Model file for the job. Use its own axes, mm. Round coordinates to 2 decimals unless told otherwise and drop trailing zeros. Write each loop counter-clockwise with the first axis right and the second up, starting at its lowest first coordinate (ties: lowest second). Pieces come first, ordered by that corner, then holes. Notation, with made-up numbers: (39.5, 30.25) - (67.5, 30.25) arc R5 cw to (67.5, 34.25) - close; hole circle Ø7 at (-19, 33). An arc over 180 degrees is marked (long way). One line per item, written item: value.
from build123d import *

# Parameters (mm, degrees)
SKETCH1_R           = 1.25
BOSS_EXTRUDE1_DEPTH = 3.9


with BuildPart() as part:
    # Sketch1 → Boss-Extrude1 (new body)
    with BuildSketch(Plane(origin=(0, 0, 0), x_dir=(1, 0, 0), z_dir=(0, 1, 0))):
        Polygon((-100, 14), (-125, 14), (-125, 5), (-121.1, 5), (-121.1, -5), (-125, -5), (-125, -14), (-60, -14), (-60, 3.5), (60, 3.5), (60, -14), (125, -14), (125, -5), (121.1, -5), (121.1, 5), (125, 5), (125, 14), (100, 14), (100, 17.9), (80, 17.9), (80, 14), (10, 14), (10, 17.9), (-10, 17.9), (-10, 14), (-80, 14), (-80, 17.9), (-100, 17.9), align=None)
        with Locations((-87.5, -9)):
            Circle(SKETCH1_R, mode=Mode.SUBTRACT)
        with Locations((87.5, -9)):
            Circle(SKETCH1_R, mode=Mode.SUBTRACT)
    extrude(amount=BOSS_EXTRUDE1_DEPTH)


solid = part.part
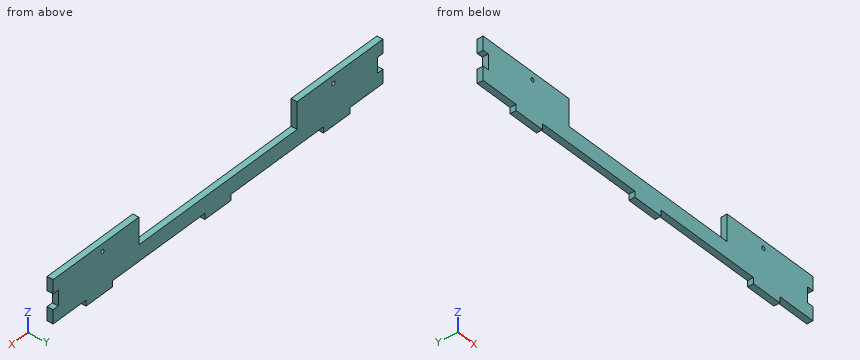
1. Band-saw the part on B-B on x = 43. Write the cut outline in (y, z), plus the area to 4 significant figures.
Report:
outline: (0, -14) - (3.9, -14) - (3.9, -3.5) - (0, -3.5) - close
area: 40.95 mm²
2. Drop flat-ended pins along their axis: pin 1 (1.2 mm diameter, centred on x = -116.5, y = 2.5, fed in from -Z); pin 2 (2 mm diameter, centred on x = -87.5, z = 9, fed in from -Y); pin 3 (5 mm diameter, centred on x = -63.5, z = -5.5, fed in from -Y); pin 4 (2 mm diameter, centred on y = 2.5, z = 0.5, fed in from +X). Give the stop position or say it passes through.
Report:
pin 1: z = -14
pin 2: through
pin 3: y = 0
pin 4: x = 121.1
3. Band-saw the part on A-A on y = 3.3. State how many separate pieces and enclosed holes the cut face has, plus the area to 3 significant figures.
Report:
separate pieces: 1
enclosed holes: 2
area: 5,050 mm²
4. Wall check: probe 1 along X at (y, z) = (0.4, 9); probe 2 along X at (y, z) = (0.2, -1); probe 3 along Z at (x, y) = (87.5, 1.85). Give the ranges that are in metal, low to high. Write a range as [from, to].
Report:
probe 1: [-125, -88.75], [-86.25, -60], [60, 86.25], [88.75, 125]
probe 2: [-121.1, -60], [60, 121.1]
probe 3: [-17.9, 7.75], [10.25, 14]
